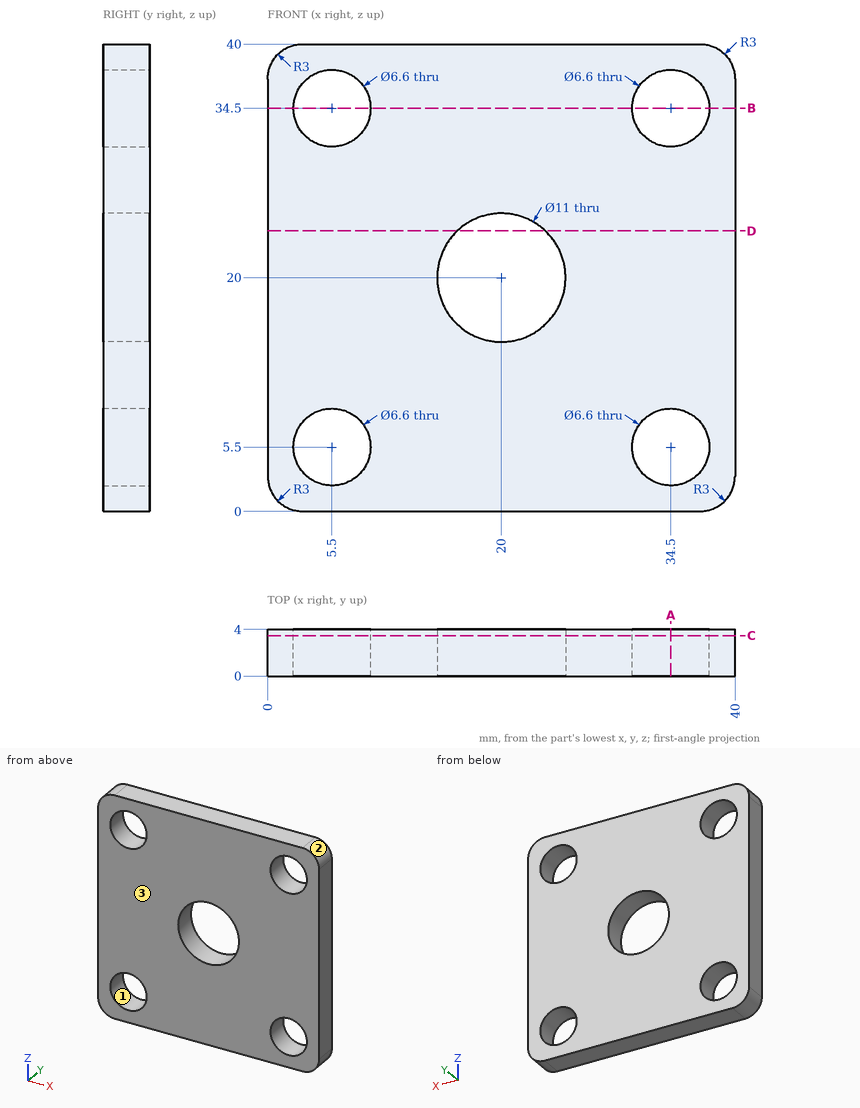
Study the drawing (mm; zero at the part's minimum x, y, z) and answer. Round coordinates to 2 decimals unless told otherwise and drop trailing zeros. Order: outer loops, then holes, each group sorted by start corner. A loop starts at its lowest first (then second) coordinate and runs counter-clockwise, first axis right, second up. Notation, with made-up numbers: (-31, 42) -> (-16, 42) arc R27 ccw to (-16, 71) -> close; hole circle Ø2 at (80, -38). An arc over 180 degrees is marked (long way). Answer as CSV lines item,"result". Start each with the question number.
(1) The part is cut by section C-C (y = 3.45). Determine the outline of the cut face in (x, z), then the cut area to 3 significant figures.
(2) Find the intervals of material crossed by probe 1 along Z at (x, y) = (34.5, 2.85); probe 2 along Z at (x, y) = (8.5, 1.6), in increasing order. Write a range as from..to.
(3) A flat-ended cylindrical pin translates along its axis: pin 1 Ø5.5 at (x, z) = (34.5, 5.5) entering from +Y. Find the tip coordinate at first contact, or state that the pin passes through.
(4) The part is cut by section A-A (x = 34.5). Determine the outline of the cut face in (y, z), then the cut area to 3 significant figures.
(5) The part is cut by section B-B (z = 34.5). Determine the outline of the cut face in (x, y).
(6) The part is cut by section D-D (z = 24). Determine the outline of the cut face in (x, y).
(7) For a pull along Z with two mould halves and no side action, classify the marked faces 1, 2 and 3 as +Z half, -Z half, draft (parallel to the pull), parting line (faces both ways), or undercut.
Evaluation:
1,outline,"(0, 3) arc R3 ccw to (3, 0) -> (37, 0) arc R3 ccw to (40, 3) -> (40, 37) arc R3 ccw to (37, 40) -> (3, 40) arc R3 ccw to (0, 37) -> close; hole circle Ø6.6 at (5.5, 5.5); hole circle Ø6.6 at (5.5, 34.5); hole circle Ø11 at (20, 20); hole circle Ø6.6 at (34.5, 5.5); hole circle Ø6.6 at (34.5, 34.5)"
1,area,"1,360 mm²"
2,probe 1,"0..2.2, 8.8..31.2, 37.8..40"
2,probe 2,"0..4.13, 6.87..33.13, 35.87..40"
3,pin 1,"through"
4,outline,"(0, 0) -> (4, 0) -> (4, 2.2) -> (0, 2.2) -> close; (0, 8.8) -> (4, 8.8) -> (4, 31.2) -> (0, 31.2) -> close; (0, 37.8) -> (4, 37.8) -> (4, 40) -> (0, 40) -> close"
4,area,"107 mm²"
5,outline,"(0, 0) -> (2.2, 0) -> (2.2, 4) -> (0, 4) -> close; (8.8, 0) -> (31.2, 0) -> (31.2, 4) -> (8.8, 4) -> close; (37.8, 0) -> (40, 0) -> (40, 4) -> (37.8, 4) -> close"
6,outline,"(0, 0) -> (16.23, 0) -> (16.23, 4) -> (0, 4) -> close; (23.77, 0) -> (40, 0) -> (40, 4) -> (23.77, 4) -> close"
7,face 1,"undercut"
7,face 2,"+Z half"
7,face 3,"draft"
